The model under review builds one solid part; all positions refer to its coordinate system, in mm. A direction names the side the tool comes from. Round coordinates to 2 decimals unless told otherwise and drop trailing zeros. Write each loop counter-clockwise with the first axis right and the second up, starting at its lowest first coordinate (ties: lowest second). Pieces come first, ordered by that corner, then holes. Notation, with made-up numbers: (86.25, 68) - (126.25, 68) arc R15 cw to (126.25, 78) - close; hole circle Ø4 at (41.5, 79). An arc over 180 degrees is marked (long way). Write each question's results on one line, items separated by ' | '.
```python
from build123d import *

# Parameters (mm, degrees)
SKETCH1_W                       = 76.8
SKETCH1_H                       = 77.4
SKETCH1_W_2                     = 72.8
SKETCH1_H_2                     = 73.25
BOSS_EXTRUDE1_DEPTH             = 3
BOSS_EXTRUDE2_REACH             = 88.454
BOSS_EXTRUDE2_DIRECTION_2_REACH = 88.454
CUT_EXTRUDE1_DEPTH              = 36.5
CUT_EXTRUDE1_DEPTH_BACK         = 36.5


with BuildPart() as part:
    # Sketch1 → Boss-Extrude1 (new body)
    with BuildSketch(Plane.XY):
        with Locations((38.4, 38.7)):
            Rectangle(SKETCH1_W, SKETCH1_H)
        with Locations((38.4, 38.7)):
            Rectangle(SKETCH1_W_2, SKETCH1_H_2, mode=Mode.SUBTRACT)
    extrude(amount=BOSS_EXTRUDE1_DEPTH)

    # Boss-Extrude2: up to this face of the body (flat: up to its plane)
    boss_extrude2_end = Plane(part.part.faces().sort_by_distance((2, 38.7, 1.5))[0])
    # Sketch3 → Boss-Extrude2 (add, up to the picked face)
    with BuildSketch(Plane.ZY.offset(-38.4), mode=Mode.PRIVATE) as boss_extrude2_sk1:
        Polygon((3, 75.325), (37.55, 75.325), (37.55, 2.075), (3, 2.075), (-11.45, 2.075), (-11.45, 75.325), align=None)
    boss_extrude2_tool1 = split(extrude(boss_extrude2_sk1.sketch, amount=BOSS_EXTRUDE2_REACH, mode=Mode.PRIVATE), bisect_by=boss_extrude2_end, keep=Keep.BOTH, mode=Mode.PRIVATE)
    add(boss_extrude2_tool1.solids().sort_by(Axis((38.4, 38.7, 13.05), (-1, 0, 0)))[0])

    # Boss-Extrude2 direction 2: up to this face of the body (flat: up to its plane)
    boss_extrude2_direction_2_end = Plane(part.part.faces().sort_by_distance((74.8, 38.7, 1.5))[0])
    # Sketch3 → Boss-Extrude2 direction 2 (add, up to the picked face)
    with BuildSketch(Plane.ZY.offset(-38.4), mode=Mode.PRIVATE) as boss_extrude2_direction_2_sk1:
        Polygon((3, 75.325), (37.55, 75.325), (37.55, 2.075), (3, 2.075), (-11.45, 2.075), (-11.45, 75.325), align=None)
    boss_extrude2_direction_2_tool1 = split(extrude(boss_extrude2_direction_2_sk1.sketch, amount=-BOSS_EXTRUDE2_DIRECTION_2_REACH, mode=Mode.PRIVATE), bisect_by=boss_extrude2_direction_2_end, keep=Keep.BOTH, mode=Mode.PRIVATE)
    add(boss_extrude2_direction_2_tool1.solids().sort_by(Axis((38.4, 38.7, 13.05), (1, 0, 0)))[0])

    # Sketch4 → Cut-Extrude1 (cut, two sides: drawn at the far end of the back side and taken through both)
    with BuildSketch(Plane.ZY.offset(-38.4).offset(-CUT_EXTRUDE1_DEPTH_BACK)):
        with BuildLine():
            Line((-10.95, 25.069274624), (-11.45, 71.427579202))
            Line((-11.45, 71.427579202), (-11.45, 2.075))
            Line((-11.45, 2.075), (-10.95, 2.075))
            Line((-10.95, 2.075), (-10.95, 24.615051172))
            Line((-10.95, 24.615051172), (-3.159893594, 24.634539463))
            ThreePointArc((-3.159893594, 24.634539463), (-1.063252525, 25.227514391), (0, 27.129360101))
            Line((0, 27.129360101), (0, 27.629360101))
            ThreePointArc((0, 27.629360101), (-1.049735735, 25.694881971), (-3.159893594, 25.069274624))
            Line((-3.159893594, 25.069274624), (-10.95, 25.069274624))
        make_face()
        with BuildLine():
            ThreePointArc((-7.449766555, 75.325), (-7.501172879, 75.325334593), (-7.552579202, 75.325))
            Line((-7.552579202, 75.325), (-7.449766555, 75.325))
        make_face()
        with BuildLine():
            Line((-11.45, 75.325), (-11.45, 71.427579202))
            ThreePointArc((-11.45, 71.427579202), (-10.293651907, 74.168651907), (-7.552579202, 75.325))
            Line((-7.552579202, 75.325), (-11.45, 75.325))
        make_face()
        with BuildLine():
            ThreePointArc((21.195514184, 26.59148761), (19.445162982, 23.729233412), (16.282917728, 22.60832602))
            Line((16.282917728, 22.60832602), (10.540023281, 22.60832602))
            Line((10.540023281, 22.60832602), (10.540023281, 2.075))
            Line((10.540023281, 2.075), (37.55, 2.075))
            Line((37.55, 2.075), (37.55, 42.945973427))
            ThreePointArc((37.55, 42.945973427), (32.588948731, 31.55253888), (21.195514184, 26.59148761))
        make_face()
        with BuildLine():
            ThreePointArc((7.633980307, 75.325), (28.610259758, 66.385259758), (37.55, 45.408980307))
            Line((37.55, 45.408980307), (37.55, 75.325))
            Line((37.55, 75.325), (7.633980307, 75.325))
        make_face()
        with BuildLine():
            Line((37.55, 45.408980307), (37.55, 44.16612845))
            ThreePointArc((37.55, 44.16612845), (37.556322242, 44.787554379), (37.55, 45.408980307))
        make_face()
        with BuildLine():
            Line((37.55, 44.16612845), (37.55, 42.945973427))
            ThreePointArc((37.55, 42.945973427), (37.560966221, 43.556050938), (37.55, 44.16612845))
        make_face()
    extrude(amount=CUT_EXTRUDE1_DEPTH + CUT_EXTRUDE1_DEPTH_BACK, mode=Mode.SUBTRACT)


solid = part.part
```
Q1. The part is to be moulded in two halves that separate along Y. For faces 5 (the flat face through (39, 22.608, 13)), 6 (the cylindrical face through (38.91, 25.71, -1.03)), 7 (the flat face through (0, 38, 1)), say which applies: released by +Y, released by -Y, zero draft, split by the parting line, or undercut.
Evaluation:
face 5: released by -Y | face 6: undercut | face 7: zero draft
Q2. We need section D-D (z = 31). State the section outline as (x, y) points.
Evaluation:
outline: (2, 30.15) - (74.8, 30.15) - (74.8, 63.7) - (2, 63.7) - close
Q3. We need section B-B (y = 18.5). State the section outline as (x, z) points, plus the area to 3 significant figures.
Evaluation:
outline: (0, 0) - (2, 0) - (2, -10.95) - (74.8, -10.95) - (74.8, 0) - (76.8, 0) - (76.8, 3) - (74.8, 3) - (74.8, 10.54) - (2, 10.54) - (2, 3) - (0, 3) - close | area: 1,580 mm^2
Q4. For probe 1 along Y at (x, z) = (12, -7.5) (3 decimals); probe 2 along Z at (x, y) = (37.5, 19.5); probe 3 along X at (y, z) = (33, 6), list the stretches that pass through material, from the lowest coordinate up.
Evaluation:
probe 1: y = 2.075 to 24.624, 25.069 to 75.325 | probe 2: z = -10.95 to 10.54 | probe 3: x = 2 to 74.8
Q5. Insertion check: P1, Ø2, axis at x = 15.5, z = -2.5, coming from the +Y side (3 decimals); P2, Ø9, axis at y = 12, z = -6.5, coming from the -X side; P3, Ø18, axis at x = 31.5, y = 9, coming from the -Z side. Each pin has a flat end and moves straight along its axis. Give the tip position at first contact, or say it passes through.
Evaluation:
P1: stops at y = 75.325 | P2: stops at x = 2 | P3: stops at z = -10.95
Q6. We need section C-C (x = 33). State the section outline as (y, z) points (3 decimals), plus the area to 3 significant figures.
Evaluation:
outline: (0, 0) - (2.075, 0) - (2.075, -10.95) - (24.615, -10.95) - (24.635, -3.16) arc R2.847 cw to (27.129, 0) - (27.629, 0) arc R2.876 ccw to (25.069, -3.16) - (25.069, -10.95) - (71.428, -11.45) arc R3.949 ccw to (75.325, -7.553) - (75.325, 0) - (77.4, 0) - (77.4, 3) - (75.325, 3) - (75.325, 7.634) arc R30.544 ccw to (45.409, 37.55) - (42.946, 37.55) arc R16.976 ccw to (26.591, 21.196) arc R5.021 ccw to (22.608, 16.283) - (22.608, 10.54) - (2.075, 10.54) - (2.075, 3) - (0, 3) - close | area: 2,680 mm^2
Q7. We need section A-A (z = -6.5). State the section outline as (x, y) points (3 decimals), plus the area to 3 significant figures.
Evaluation:
outline: (2, 2.075) - (74.8, 2.075) - (74.8, 24.626) - (2, 24.626) - close; (2, 25.069) - (74.8, 25.069) - (74.8, 75.325) - (2, 75.325) - close | area: 5,300 mm^2
Q8. Tool access review of faces 1 (the flat face through (39, 75.325, -4)), 2 (the flat face through (39, 2.075, -6)), 3 (the cylindrical face through (38.9, 25.2, -1.1)), 4 (the flat face through (2, 14, -5)): name each direction out of +Z, -Z, +X, -X, +Y, -Y from which nothing blocks a thin tool from reaching the whole face with its end or side.
Evaluation:
face 1: -Z, +X, -X, +Y | face 2: -Z, +X, -X, -Y | face 3: +X, -X | face 4: -Z, -X, +Y, -Y
